Source: CAD feature listing. Evaluate the final solid. Frame: model axes, mm. A direction names the side the tool comes from. Give positions to 0.01 mm unless a question says otherwise; leave off trailing zeros. Order: outer loops, then holes, each group sorted by start corner. A loop starts at its lowest first (then second) coordinate and runs counter-clockwise, first axis right, second up. Notation, with made-up numbers: (-1, 21.5) - (27, 21.5) arc R16 ccw to (27, 52.5) - close; hole circle Ø2 at (-10.5, 11). An arc over 180 degrees is marked (long way). Use CSV: the item, a comma, the result in double quotes.
```python
from build123d import *

# Parameters (mm, degrees)
ESTRUSIONE_ESTRUSIONE2_DEPTH = 12.55
ESTRUSIONE_ESTRUSIONE3_DEPTH = 3.5
ESTRUSIONE_ESTRUSIONE4_DEPTH = 1.3
SCHIZZO4_R                   = 2.35
SCHIZZO4_R_2                 = 0.85
ESTRUSIONE_ESTRUSIONE5_DEPTH = 3
TAGLIO_ESTRUSIONE1_REACH     = 30.477
SCHIZZO6_R                   = 1.5


with BuildPart() as part:
    # Schizzo1 → Estrusione-Estrusione2 (new body)
    with BuildSketch(Plane.XY):
        Polygon((11.4, 21.717893219), (12.867893219, 20.25), (15.6, 20.25), (15.6, 18.8), (11.4, 18.8), (11.4, 0), (-11.4, 0), (-11.4, 18.8), (-15.6, 18.8), (-15.6, 20.25), (-12.867893219, 20.25), (-11.4, 21.717893219), (-11.4, 24.6), (11.4, 24.6), align=None)
    extrude(amount=ESTRUSIONE_ESTRUSIONE2_DEPTH)

    # Schizzo2 → Estrusione-Estrusione3 (add)
    with BuildSketch(Plane(origin=(0, 24.6, 0), x_dir=(1, 0, 0), z_dir=(0, 1, 0))):
        with BuildLine():
            Line((0.6, -3.125), (-0.293386641, -3.125))
            ThreePointArc((-0.293386641, -3.125), (-11.4, -6.275), (-0.293386641, -9.425))
            Line((-0.293386641, -9.425), (0.6, -9.425))
            ThreePointArc((0.6, -9.425), (3.75, -6.275), (0.6, -3.125))
        make_face()
    extrude(amount=ESTRUSIONE_ESTRUSIONE3_DEPTH)

    # Schizzo3 → Estrusione-Estrusione4 (add)
    with BuildSketch(Plane(origin=(0, 28.1, 0), x_dir=(1, 0, 0), z_dir=(0, 1, 0))):
        with BuildLine():
            Line((-0.885855563, -8.425), (0.6, -8.425))
            ThreePointArc((0.6, -8.425), (2.75, -6.275), (0.6, -4.125))
            Line((0.6, -4.125), (-0.885855563, -4.125))
            ThreePointArc((-0.885855563, -4.125), (-10.4, -6.275), (-0.885855563, -8.425))
        make_face()
    extrude(amount=ESTRUSIONE_ESTRUSIONE4_DEPTH)

    # Schizzo4 → Estrusione-Estrusione5 (add)
    with BuildSketch(Plane(origin=(0, 29.4, 0), x_dir=(1, 0, 0), z_dir=(0, 1, 0))):
        with Locations(Location((-5.4, -6.275, 0), (0, 0, 270))):
            Circle(SCHIZZO4_R)
        with Locations(Location((-5.4, -6.275, 0), (0, 0, 270))):
            Circle(SCHIZZO4_R_2, mode=Mode.SUBTRACT)
    extrude(amount=ESTRUSIONE_ESTRUSIONE5_DEPTH)

    # Schizzo6 → Taglio-Estrusione1 (cut, up to next)
    with BuildSketch(Plane(origin=(0, 20.25, 0), x_dir=(1, 0, 0), z_dir=(0, 1, 0)), mode=Mode.PRIVATE) as taglio_estrusione1_sk1:
        with Locations((-14.867893219, -6.275)):
            Circle(SCHIZZO6_R)
    taglio_estrusione1_tool1 = extrude(taglio_estrusione1_sk1.sketch, amount=-TAGLIO_ESTRUSIONE1_REACH, mode=Mode.PRIVATE) & part.part
    # Schizzo6 → Taglio-Estrusione1 (cut, up to next)
    with BuildSketch(Plane(origin=(0, 20.25, 0), x_dir=(1, 0, 0), z_dir=(0, 1, 0)), mode=Mode.PRIVATE) as taglio_estrusione1_sk2:
        with Locations((14.867893219, -6.275)):
            Circle(SCHIZZO6_R)
    taglio_estrusione1_tool2 = extrude(taglio_estrusione1_sk2.sketch, amount=-TAGLIO_ESTRUSIONE1_REACH, mode=Mode.PRIVATE) & part.part
    add(taglio_estrusione1_tool1.solids().sort_by_distance((-14.867893, 20.25, 6.275))[0], mode=Mode.SUBTRACT)
    add(taglio_estrusione1_tool2.solids().sort_by_distance((14.867893, 20.25, 6.275))[0], mode=Mode.SUBTRACT)


solid = part.part
```
Item 1: Section C-C on z = 2. Return the cut outline in (x, y).
Filled in:
outline,"(-15.6, 18.8) - (-11.4, 18.8) - (-11.4, 0) - (11.4, 0) - (11.4, 18.8) - (15.6, 18.8) - (15.6, 20.25) - (12.87, 20.25) - (11.4, 21.72) - (11.4, 24.6) - (-1.19, 24.6) - (-1.19, 28.1) - (-2.81, 28.1) - (-2.81, 29.4) - (-7.99, 29.4) - (-7.99, 28.1) - (-9.61, 28.1) - (-9.61, 24.6) - (-11.4, 24.6) - (-11.4, 21.72) - (-12.87, 20.25) - (-15.6, 20.25) - close"
Item 2: First-contact query: pin 1 (4 mm diameter, centred on y = 8, z = 8, fed in from +X); pin 2 (1.3 mm diameter, centred on x = 13.5, z = 6, fed in from -Y); pin 3 (4 mm diameter, centred on x = 5.5, z = 8.5, fed in from +Y). Flat tips, straight axial feed; report the tip coordinate or a pass-through.
Filled in:
pin 1,"stops at x = 11.4"
pin 2,"stops at y = 18.8"
pin 3,"stops at y = 24.6"
Item 3: Section B-B on y = 14. Return the cut outline in (x, z), then the cut area to 3 significant figures.
Filled in:
outline,"(-11.4, 0) - (11.4, 0) - (11.4, 12.55) - (-11.4, 12.55) - close"
area,"286 mm2"
Item 4: Set-up query: faces 1 (the flat face through (-13, 18.8, 6)), 2 (the flat face through (-13.04, 20.25, 6.19)), 3 (the cylindrical face through (2.75, 28.74, 6.32)). Return all of +Z, -Z, +X, -X, +Y, -Y with unobstructed straight access to the full face (end or side cutting, diameter ignored); none if empty.
Filled in:
face 1,"+Z, -Z, -X, -Y"
face 2,"+Z, -Z, -X, +Y"
face 3,"+X, +Y"
Item 5: Section A-A on x = -5.4. Return the cut outline in (y, z) (3 decimals).
Filled in:
outline,"(0, 0) - (24.6, 0) - (24.6, 0.275) - (28.1, 0.275) - (28.1, 1.275) - (29.4, 1.275) - (29.4, 3.925) - (32.4, 3.925) - (32.4, 5.425) - (29.4, 5.425) - (29.4, 7.125) - (32.4, 7.125) - (32.4, 8.625) - (29.4, 8.625) - (29.4, 11.275) - (28.1, 11.275) - (28.1, 12.275) - (24.6, 12.275) - (24.6, 12.55) - (0, 12.55) - close"
Item 6: Section D-D on y = 29. Return the cut outline in (x, z) (3 decimals).
Filled in:
outline,"(-0.886, 4.125) - (0.6, 4.125) arc R2.15 ccw to (0.6, 8.425) - (-0.886, 8.425) arc R5 ccw (long way) to start"
Item 7: Material intervals for line 1 (X direction, y = 11, z = 4.5); line 2 (Y direction, x = 4.5, z = 1.75); line 3 (Z direction, x = -5, y = 31) (3 decimals), sorted ascending. Write a range as from..to.
Filled in:
line 1,"x = -11.4..11.4"
line 2,"y = 0..24.6"
line 3,"z = 3.959..5.525, 7.025..8.591"
